```python
from build123d import *

# Parameters (mm, degrees)
VYSUNOUT1_DEPTH = 1.25
SKICA4_R        = 3
VYSUNOUT2_DEPTH = 4.5
ZKOSIT1_SIZE    = 0.5


with BuildPart() as part:
    # Skica1 → Vysunout1 (new, symmetric)
    with BuildSketch(Plane.XY):
        Polygon((4.041451884, 0), (2.020725942, 3.5), (-2.020725942, 3.5), (-4.041451884, 0), (-2.020725942, -3.5), (2.020725942, -3.5), align=None)
    extrude(amount=VYSUNOUT1_DEPTH, both=True)

    # Skica2 → Odebrat otočením1 (revolve, cut)
    with BuildSketch(Plane(origin=(0, 0, 0), x_dir=(0, 0, -1), z_dir=(1, 0, 0))):
        Polygon((-1.25, 3.5), (-1.25, 5.142284655), (-0.301826512, 5.142284655), align=None)
    odebrat_oto_en_m1 = revolve(axis=Axis((0, 0, 1.25), (0, 0, 1)), mode=Mode.SUBTRACT)

    # Zrcadlit1: Odebrat otočením1 across plane
    add(odebrat_oto_en_m1.mirror(Plane.XY), mode=Mode.SUBTRACT)

    # Skica3 → Otočit kolem osy1 (revolve)
    with BuildSketch(Plane(origin=(0, 0, 0), x_dir=(0, 0, -1), z_dir=(1, 0, 0)), mode=Mode.PRIVATE) as oto_it_kolem_osy1_sk:
        with BuildLine():
            Line((-8.75, 1.65), (-8.75, 0))
            Line((-8.75, 0), (-1.25, 0))
            Line((-1.25, 0), (-1.25, 3.25))
            ThreePointArc((-1.25, 3.25), (-1.33004432, 2.978638199), (-1.544548907, 2.794160282))
            ThreePointArc((-1.544548907, 2.794160282), (-2.686883352, 2.472411814), (-3.873344034, 2.5))
            ThreePointArc((-3.873344034, 2.5), (-6.508060613, 3.201728963), (-8.75, 1.65))
        make_face()
    revolve(oto_it_kolem_osy1_sk.sketch.rotate(Axis((0, 0, 1.25), (0, 0, -1)), 180), axis=Axis((0, 0, 1.25), (0, 0, -1)))

    # Skica4 → Vysunout2 (add)
    with BuildSketch(Plane(origin=(0, 0, -1.25), x_dir=(-1, 0, 0), z_dir=(0, 0, -1))):
        Circle(SKICA4_R)
    extrude(amount=VYSUNOUT2_DEPTH)

    # Zkosit1
    zkosit1_edges = [part.edges().sort_by_distance(p)[0] for p in [
        (3, 0, -5.75),
    ]]
    chamfer(zkosit1_edges, length=ZKOSIT1_SIZE)


solid = part.part
```
Source: CAD feature listing. Evaluate the final solid. Frame: model axes, mm. Coordinates: 2 decimals unless noted, no trailing zeros. Write each loop counter-clockwise with the first axis right and the second up, starting at its lowest first coordinate (ties: lowest second). Pieces come first, ordered by that corner, then holes. Notation, with made-up numbers: (89.25, -15.5) - (116.25, -15.5) arc R23 ccw to (116.25, -5.5) - close; hole circle Ø8 at (78.5, -1.75). An arc over 180 degrees is marked (long way). Answer as a JSON object with one key per item and string values.
Q1. Section query A-A, the plane z = -4.5. Output: boundary loops of the cut face in (x, y).
Ans:
{"outline": "circle Ø6 at (0, 0)"}
Q2. First-contact query: pin 1 Ø4 at (x, z) = (1, 4) entering from +Y. Flat tip, straight axial feed; report the tip coordinate or a pass-through.
Ans:
{"pin 1": "stops at y = 3.24"}
Q3. Material intervals for line 1 (Z direction, x = 2.25, y = -2.5); line 2 (X direction, y = 0.5, z = 7); line 3 (X direction, y = 2.75, z = 5.5), sorted ascending. Write a range as [from, to].
Ans:
{"line 1": "z = [-1.25, 1.25]", "line 2": "x = [-3.03, 3.03]", "line 3": "x = [-1.67, 1.67]"}
Q4. Section query B-B, the plane z = 2.75. Output: boundary loops of the cut face in (x, y).
Ans:
{"outline": "circle Ø4.93 at (0, 0)"}
Q5. Draft query along X for faces 1 (the flat face through (3, 1, -1.25)), 2 (the conical face through (3.69, -0.01, 1.14)), 3 (the cylindrical face through (3, 0, -3)), 4 (the conical face through (-1.85, -3.19, -1.14)). Return one class per face: released by +X, released by -X, zero draft, split by the parting line, or undercut.
Ans:
{"face 1": "zero draft", "face 2": "released by +X", "face 3": "split by the parting line", "face 4": "released by -X"}
